Could you check a few things on this model? Use its own coordinates, in mm. Face numbers are marked on the shaded views. Coordinates: 2 decimals unless noted, no trailing zeros. Write each loop counter-clockwise with the first axis right and the second up, starting at its lowest first coordinate (ties: lowest second). Pieces come first, ordered by that corner, then holes.
Item 1: I want a section at C-C on z = 6. Please give me the cut outline in (x, y), then the cut area to 3 significant figures.
Item 2: If I drill on probe 1 along X at (y, z) = (-10.5, 16.6); probe 2 along Y at (x, z) = (-0.5, 16.3); probe 3 along Y at (x, z) = (2, 8), over which ranges is the centre line in solid material (lowest first)?
Item 3: I want a section at A-A on y = -10.5. Please give me the cut outline in (x, z).
Item 4: I want a section at D-D on y = 28.5. Please give me the cut outline in (x, z), then the cut area to 3 significant figures.
Item 5: Thinking about a two-plate mould opening in X: for the marked faces 1 and 2, which applies, +X half, -X half, draft (parallel to the pull), parting line (faces both ways), or undercut?
Item 6: For P1, Ø1.6, axis at x = -0.5, y = -10.5, coming from the -Z side; P2, Ø12, axis at x = 27.5, y = 12.5, coming from the -Z side; P3, Ø3.5, axis at x = 29.86, y = 62.23, coming from the +Z side; P4, Ø1, axis at y = 2, z = 5, coming from the -X side, each with a flat end and sliding along its axis, tell me the tip position at first contact or that it passes through.
Item 7: I want a section at B-B on x = 3.5. Please give me the cut outline in (y, z).
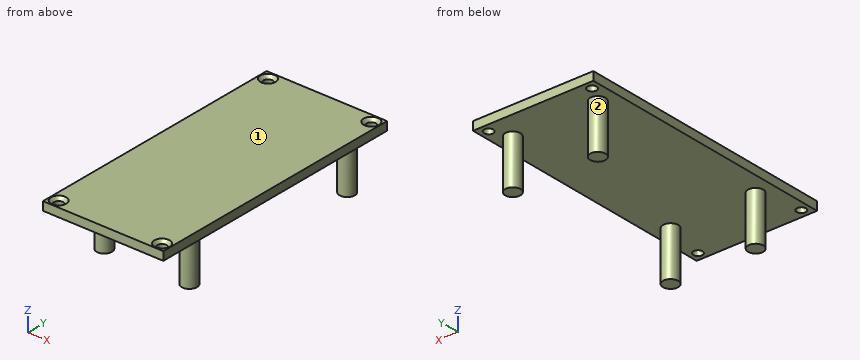
from build123d import *

# Parameters (mm, degrees)
SKETCH009_W      = 35.3624
SKETCH009_H      = 77.7328
PAD004_DEPTH     = 2.5
SKETCH010_R      = 2.25
PAD005_DEPTH     = 14.4
HOLE_D           = 2.7
HOLE_CSINK_D     = 4.5
HOLE_CSINK_ANGLE = 90


with BuildPart() as part:
    # Sketch009 (on CopyDatumPlane) → Pad004 (new body)
    with BuildSketch(Plane.XY.offset(16)):
        with Locations((14.6812, 25.8664)):
            Rectangle(SKETCH009_W, SKETCH009_H)
    extrude(amount=PAD004_DEPTH)

    # Sketch010 (on CopyDatumPlane) → Pad005 (join)
    with BuildSketch(Plane.XY.offset(16)):
        with Locations((2.1844, 57.038)):
            Circle(SKETCH010_R)
        with Locations((27.178, 57.038)):
            Circle(SKETCH010_R)
        with Locations((27.178, 2.174)):
            Circle(SKETCH010_R)
        with Locations((2.1844, 2.174)):
            Circle(SKETCH010_R)
    extrude(amount=-PAD005_DEPTH)

    # Hole (through all)
    with Locations(Plane.XY.offset(18.5)):
        with Locations((-0.5, 62.2328), (29.8624, 62.2328), (29.8624, -10.5), (-0.5, -10.5)):
            CounterSinkHole(HOLE_D / 2, HOLE_CSINK_D / 2, counter_sink_angle=HOLE_CSINK_ANGLE)


solid = part.part
Response values:
1. outline: circle Ø4.5 at (2.18, 2.17); circle Ø4.5 at (2.18, 57.04); circle Ø4.5 at (27.18, 2.17); circle Ø4.5 at (27.18, 57.04)
1. area: 63.6 mm2
2. probe 1: x = -3 to -1.85, 0.85 to 28.51, 31.21 to 32.36
2. probe 2: y = -13 to -11.85, -9.15 to 60.88, 63.58 to 64.73
2. probe 3: y = -0.07 to 4.42, 54.8 to 59.28
3. outline: (-3, 16) - (-1.85, 16) - (-1.85, 17.6) - (-2.75, 18.5) - (-3, 18.5) - close; (0.85, 16) - (28.51, 16) - (28.51, 17.6) - (27.61, 18.5) - (1.75, 18.5) - (0.85, 17.6) - close; (31.21, 16) - (32.36, 16) - (32.36, 18.5) - (32.11, 18.5) - (31.21, 17.6) - close
4. outline: (-3, 16) - (32.36, 16) - (32.36, 18.5) - (-3, 18.5) - close
4. area: 88.4 mm2
5. face 1: draft
5. face 2: undercut
6. P1: passes through
6. P2: stops at z = 16
6. P3: stops at z = 18
6. P4: stops at x = -0.07
7. outline: (-13, 16) - (0.35, 16) - (0.35, 1.6) - (4, 1.6) - (4, 16) - (55.21, 16) - (55.21, 1.6) - (58.86, 1.6) - (58.86, 16) - (64.73, 16) - (64.73, 18.5) - (-13, 18.5) - close
